Geometry check sheet. Reference: the model listing, model coordinates, mm. A direction names the side the tool comes from. Coordinates: 2 decimals unless noted, no trailing zeros. Write each loop counter-clockwise with the first axis right and the second up, starting at its lowest first coordinate (ties: lowest second). Pieces come first, ordered by that corner, then holes.
from build123d import *

# Parameters (mm, degrees)
SKETCH_1_W      = 55
SKETCH_1_H      = 40
SKETCH_1_W_2    = 45
SKETCH_1_H_2    = 30
SKETCH_1_W_3    = 16
SKETCH_1_H_3    = 5
EXTRUDE_1_DEPTH = 5
FILLET_1_R      = 10
FILLET_2_R      = 15
EXTRUDE_START   = -5
SKETCH_2_W      = 5
SKETCH_2_H      = 7
EXTRUDE_2_DEPTH = 5.01
FILLET_3_R      = 15


with BuildPart() as part:
    # ｽｹｯﾁ1 → ﾎﾞｽ - 押し出し1 (new body)
    # profile 1 of 3: a face of its own
    with BuildSketch(Plane.XY):
        with Locations((35.5, 1.53340789)):
            Rectangle(SKETCH_1_W, SKETCH_1_H)
        with Locations((35.5, 1.53340789)):
            Rectangle(SKETCH_1_W_2, SKETCH_1_H_2, mode=Mode.SUBTRACT)
    # profile 2 of 3: a face of its own
    with BuildSketch(Plane.XY):
        with Locations((0, 19.03340789)):
            Rectangle(SKETCH_1_W_3, SKETCH_1_H_3)
    # profile 3 of 3: a face of its own
    with BuildSketch(Plane.XY):
        with Locations((-35.5, 1.53340789)):
            Rectangle(SKETCH_1_W, SKETCH_1_H)
        with Locations((-35.5, 1.53340789)):
            Rectangle(SKETCH_1_W_2, SKETCH_1_H_2, mode=Mode.SUBTRACT)
    extrude_1 = extrude(amount=EXTRUDE_1_DEPTH)

    # ﾌｨﾚｯﾄ1
    fillet_1_edges = [part.edges().sort_by_distance(p)[0] for p in [
        (-58, -13.46659211, 2.5),
        (-13, -13.46659211, 2.5),
        (13, -13.46659211, 2.5),
        (58, -13.46659211, 2.5),
    ]]
    fillet(fillet_1_edges, radius=FILLET_1_R)

    # ﾌｨﾚｯﾄ2
    fillet_2_edges = [part.edges().sort_by_distance(p)[0] for p in [
        (63, -18.46659211, 2.5),
        (8, -18.46659211, 2.5),
        (-8, -18.46659211, 2.5),
        (-63, -18.46659211, 2.5),
    ]]
    fillet(fillet_2_edges, radius=FILLET_2_R)

    # ｽｹｯﾁ2 → ﾎﾞｽ - 押し出し2 (add)
    with BuildSketch(Plane.ZY.offset(63).offset(EXTRUDE_START)):
        with Locations((2.5, 18.03340789)):
            Rectangle(SKETCH_2_W, SKETCH_2_H)
        Polygon((87.451237669, 15.948400854), (91.671154304, 21.53340789), (5, 21.53340789), (5, 14.53340789), (89.323963209, 14.53340789), align=None)
        Polygon((91.671154304, 14.53340789), (91.671154304, 21.53340789), (87.451237669, 15.948400854), (89.323963209, 14.53340789), align=None)
        Polygon((110, 7.684508442), (91.671154304, 21.53340789), (91.671154304, 14.53340789), (89.323963209, 14.53340789), (105.780083365, 2.099501406), align=None)
    extrude_2 = extrude(amount=EXTRUDE_2_DEPTH)

    # ﾐﾗｰ1: ﾎﾞｽ - 押し出し1, ﾎﾞｽ - 押し出し2 across plane
    add(extrude_1.mirror(Plane(origin=(0, 0, 0), x_dir=(0, 0, 1), z_dir=(1, 0, 0))))
    add(extrude_2.mirror(Plane(origin=(0, 0, 0), x_dir=(0, 0, 1), z_dir=(1, 0, 0))))

    # ﾌｨﾚｯﾄ3
    fillet_3_edges = [part.edges().sort_by_distance(p)[0] for p in [
        (63, -18.46659211, 2.5),
        (-8, -18.46659211, 2.5),
        (-63, -18.46659211, 2.5),
        (8, -18.46659211, 2.5),
    ]]
    fillet(fillet_3_edges, radius=FILLET_3_R)


solid = part.part
1. Sectioned sample at C-C, the plane x = -41. Record the boundary of the cut face in (y, z), and give its area (3 significant figures).
Computed values:
outline: (-18.47, 0) - (-13.47, 0) - (-13.47, 5) - (-18.47, 5) - close; (16.53, 0) - (21.53, 0) - (21.53, 5) - (16.53, 5) - close
area: 50.0 mm2
2. Gauge pin test, flat ends, axial feed: pin 1 Ø2.5 at (x, z) = (61, 24.5) entering from -Y; pin 2 Ø1.5 at (y, z) = (5.5, 3.5) entering from -X; pin 3 Ø2.5 at (y, z) = (3.5, 3) entering from +X. Record the tip position at first contact, or that the pin passes through.
Computed values:
pin 1: stops at y = 14.53
pin 2: stops at x = -63
pin 3: stops at x = 63
3. Thickness scan on line 1 along Z through (x, y) = (12.5, 5). Record the ranges inside material, lowest first.
Computed values:
line 1: z = 0 to 5
4. Access from +Z, -Z, +X, -X, +Y, -Y to the whole of each face (thin tool, end or side, straight path). Record for faces 4 (the flat face through (60.47, 8.4, 97.44)), 5 (the flat face through (0, 16.533, 2)), 6 (the cylindrical face through (-15.85, -10.46, 2.54)), 7 (the flat face through (-9, 2, 0)), 8 (the flat face through (35, -18.467, 2)).
Computed values:
face 4: +X, -X, -Y
face 5: +Z, -Z, -Y
face 6: +Z, -Z
face 7: -Z, +X, -X, +Y, -Y
face 8: +Z, -Z, +X, -X, -Y
5. Sectioned sample at D-D, the plane y = -11. Record the boundary of the cut face in (x, z).
Computed values:
outline: (-60.97, 0) - (-54.58, 0) - (-54.58, 5) - (-60.97, 5) - close; (-16.42, 0) - (-10.03, 0) - (-10.03, 5) - (-16.42, 5) - close; (10.03, 0) - (16.42, 0) - (16.42, 5) - (10.03, 5) - close; (54.58, 0) - (60.97, 0) - (60.97, 5) - (54.58, 5) - close
6. Draft check along Y on faces 1 (the flat face through (-60, 14.533, 44)), 2 (the cylindrical face through (-55.15, -10.46, 2.54)), 3 (the flat face through (0, 21.533, 1)). Enter one of: released by +Y, released by -Y, zero draft, split by the parting line, or undercut.
Computed values:
face 1: released by -Y
face 2: undercut
face 3: released by +Y
7. Sectioned sample at A-A, the plane z = 10. Record the boundary of the cut face in (x, y), and give its area (3 significant figures).
Computed values:
outline: (-63.01, 14.53) - (-58, 14.53) - (-58, 21.53) - (-63.01, 21.53) - close; (58, 14.53) - (63.01, 14.53) - (63.01, 21.53) - (58, 21.53) - close
area: 70.1 mm2
8. Sectioned sample at B-B, the plane y = 5. Record the boundary of the cut face in (x, z).
Computed values:
outline: (-63.01, 101.94) - (-58, 101.94) - (-58, 107.97) - (-63.01, 107.97) - close; (-63, 0) - (-58, 0) - (-58, 5) - (-63, 5) - close; (-13, 0) - (-8, 0) - (-8, 5) - (-13, 5) - close; (8, 0) - (13, 0) - (13, 5) - (8, 5) - close; (58, 0) - (63, 0) - (63, 5) - (58, 5) - close; (58, 101.94) - (63.01, 101.94) - (63.01, 107.97) - (58, 107.97) - close
